Design review of the part built by this model. Coordinates are the model's own, in mm. A direction names the side the tool comes from. Coordinates: 2 decimals unless noted, no trailing zeros. Write each loop counter-clockwise with the first axis right and the second up, starting at its lowest first coordinate (ties: lowest second). Pieces come first, ordered by that corner, then holes.
Q1. Machinability: for faces 1 (the face through (-18.75, 0, -1)), 2 (the face through (17.95, 0, 5)), 3 (the face through (21, 10, 5)), 4 (the face through (0, 16, -1)), 5 (the face through (18.75, 0, -1)), which of the approach directions +Z, -Z, +X, -X, +Y, -Y give a long, thin tool a straight path to every point of the face, cutting with its end or side? Answer none if there is none.
Q2. Add section B-B, the plane y = 8. Give the boundary of the cut face in (x, z), plus the area to 3 significant figures.
Q3. The part is to be moulded in two halves that separate along Y. For faces 6 (the face through (0, 16.5, 1)), 7 (the face through (20.02, -14.45, 0.79)), 8 (the face through (21, -10, 5)), say which applies: +Y half, -Y half, draft (parallel to the pull), parting line (faces both ways), or undercut.
Q4. Clearance check with flat-ended pins moving along their axes: pin 1 Ø3.5 at (x, y) = (21.45, -14) entering from +Z; pin 2 Ø16.5 at (x, y) = (-1, 1) entering from -Z; pin 3 Ø3 at (y, z) = (-4.5, 5.5) entering from -X. State where each tip first meets the part, or that it passes through.
Q5. Add section D-D, the plane z = 2.5. Give the boundary of the cut face in (x, y), plus the area to 3 significant figures.
Q6. Add section A-A, the plane x = 21.45. Give the boundary of the cut face in (y, z).
Q7. To check wall thickness, follow probe 1 along Y at (x, z) = (21.45, 0.45); probe 2 along Z at (x, y) = (7.5, 1); probe 3 along X at (y, z) = (4, 5). State the ranges of each line that lie inside material, in increasing order.
Q8. Add section C-C, the plane x = -21.45. Give the boundary of the cut face in (y, z), plus the area to 3 significant figures.
from build123d import *

# Parameters (mm, degrees)
BASE_PCB_2_W              = 47.9
BASE_PCB_2_H              = 33
BASE_PCB_2_R              = 1.5
BASE_PCB_DEPTH            = 1.6
ESQUISSE4_W               = 37.5
ESQUISSE4_H               = 32
E_INK_DISPLAY_DEPTH       = 1.2
ESQUISSE5_W               = 27.6
ESQUISSE5_H               = 27.6
DISPLAY_200_200_DEPTH     = 0.5
ESQUISSE6_W               = 6
ESQUISSE6_H               = 20
CONNECTEUR_8BROCHES_DEPTH = 6


with BuildPart() as part:
    # BASE PCB 2 → Base_PCB (new body)
    with BuildSketch(Plane.XY):
        Rectangle(BASE_PCB_2_W, BASE_PCB_2_H)
        with Locations((-21.45, 14)):
            Circle(BASE_PCB_2_R, mode=Mode.SUBTRACT)
        with Locations((-21.45, -14)):
            Circle(BASE_PCB_2_R, mode=Mode.SUBTRACT)
        with Locations(Location((21.45, -14, 0), (0, 0, 180))):
            Circle(BASE_PCB_2_R, mode=Mode.SUBTRACT)
        with Locations(Location((21.45, 14, 0), (0, 0, 180))):
            Circle(BASE_PCB_2_R, mode=Mode.SUBTRACT)
    extrude(amount=BASE_PCB_DEPTH)

    # Esquisse4 → E-Ink_display (add)
    with BuildSketch(Plane.XY):
        Rectangle(ESQUISSE4_W, ESQUISSE4_H)
    extrude(amount=-E_INK_DISPLAY_DEPTH)

    # Esquisse5 → Display_200*200 (cut)
    with BuildSketch(Plane(origin=(0, 0, -1.2), x_dir=(-1, 0, 0), z_dir=(0, 0, -1))):
        with Locations((-2.95, 0)):
            Rectangle(ESQUISSE5_W, ESQUISSE5_H)
    extrude(amount=-DISPLAY_200_200_DEPTH, mode=Mode.SUBTRACT)

    # Esquisse6 → Connecteur_8broches (add)
    with BuildSketch(Plane.XY.offset(1.6)):
        with Locations((20.95, 0)):
            Rectangle(ESQUISSE6_W, ESQUISSE6_H)
    extrude(amount=CONNECTEUR_8BROCHES_DEPTH)


solid = part.part
Here are the results:
1. face 1: -Z, -X, +Y, -Y
1. face 2: +Z, -X, +Y, -Y
1. face 3: +Z, +X, -X, +Y
1. face 4: -Z, +X, -X, +Y
1. face 5: -Z, +X, +Y, -Y
2. outline: (-23.95, 0) - (-18.75, 0) - (-18.75, -1.2) - (-10.85, -1.2) - (-10.85, -0.7) - (16.75, -0.7) - (16.75, -1.2) - (18.75, -1.2) - (18.75, 0) - (23.95, 0) - (23.95, 7.6) - (17.95, 7.6) - (17.95, 1.6) - (-23.95, 1.6) - close
2. area: 144 mm2
3. face 6: +Y half
3. face 7: undercut
3. face 8: -Y half
4. pin 1: stops at z = 1.6
4. pin 2: stops at z = -0.7
4. pin 3: stops at x = 17.95
5. outline: (17.95, -10) - (23.95, -10) - (23.95, 10) - (17.95, 10) - close
5. area: 120 mm2
6. outline: (-16.5, 0) - (-15.5, 0) - (-15.5, 1.6) - (-16.5, 1.6) - close; (-12.5, 0) - (12.5, 0) - (12.5, 1.6) - (10, 1.6) - (10, 7.6) - (-10, 7.6) - (-10, 1.6) - (-12.5, 1.6) - close; (15.5, 0) - (16.5, 0) - (16.5, 1.6) - (15.5, 1.6) - close
7. probe 1: y = -16.5 to -15.5, -12.5 to 12.5, 15.5 to 16.5
7. probe 2: z = -0.7 to 1.6
7. probe 3: x = 17.95 to 23.95
8. outline: (-16.5, 0) - (-15.5, 0) - (-15.5, 1.6) - (-16.5, 1.6) - close; (-12.5, 0) - (12.5, 0) - (12.5, 1.6) - (-12.5, 1.6) - close; (15.5, 0) - (16.5, 0) - (16.5, 1.6) - (15.5, 1.6) - close
8. area: 43.2 mm2
